```python
from build123d import *

# Parameters (mm, degrees)
F0_R     = 11.5
F0_R_2   = 5.5
F1_DEPTH = 1
F0_R_3   = 4.05
F2_DEPTH = 2
F0_R_4   = 2
F3_DEPTH = 5


# Not quite as in the source:
# - a fillet or chamfer that OpenCascade refuses, or shapes differently, is made with other operations: its cross-section is extruded or revolved along the edge and cut away or added


with BuildPart() as f1:
    # F0 (on Top) → F1 (new body)
    with BuildSketch(Plane.XY):
        Circle(F0_R)
        Circle(F0_R_2, mode=Mode.SUBTRACT)
    extrude(amount=F1_DEPTH)

    # F0 (on Top) → F2 (join)
    with BuildSketch(Plane.XY):
        Circle(F0_R_2)
        Circle(F0_R_3, mode=Mode.SUBTRACT)
    extrude(amount=F2_DEPTH)

    # F0 (on Top) → F3 (join)
    with BuildSketch(Plane.XY):
        Circle(F0_R_3)
        Circle(F0_R_4, mode=Mode.SUBTRACT)
        Circle(F0_R_4)
    extrude(amount=F3_DEPTH)

    # F4: fillet of radius 2 on 1 edges, made by hand

    # F4_s1 → F4_t2 (revolve, cut)
    with BuildSketch(Plane.XZ):
        with BuildLine():
            ThreePointArc((11.5, 1), (10.7679491924, 0.2679491924), (9.7679491924, 0))
            Line((9.7679491924, 0), (11.5, 0))
            Line((11.5, 0), (11.5, 1))
        make_face()
    revolve(axis=Axis((0, 0, 0), (0, 0, 1)), mode=Mode.SUBTRACT)


solid = f1.part
```
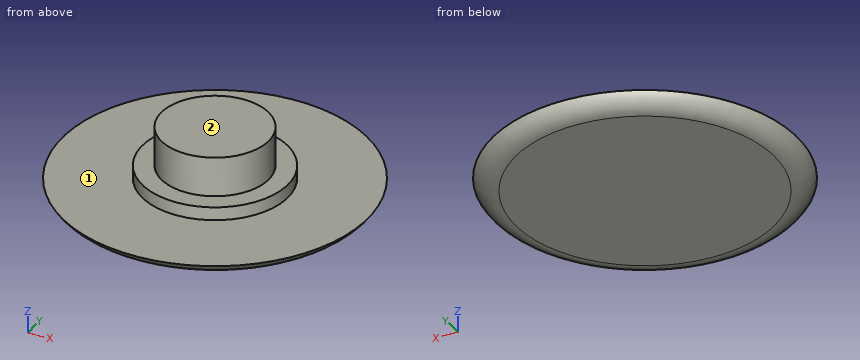
Geometry: final body of the model. Coordinates: model frame, mm. Face numbers are marked on the shaded views. A direction names the side the tool comes from. Coordinates: 2 decimals unless noted, no trailing zeros. Order: outer loops, then holes, each group sorted by start corner. A loop starts at its lowest first (then second) coordinate and runs counter-clockwise, first axis right, second up. Notation, with made-up numbers: (-7.75, 40.5) - (12.25, 40.5) arc R16 ccw to (12.25, 54.5) - close; hole circle Ø9 at (-1.75, 46.5). An arc over 180 degrees is marked (long way). Write each question's results on one line, items separated by ' | '.
1) Section C-C, the plane z = 2.8. Return loops of the section in (x, y), plus the area to 3 significant figures.
Results list:
outline: circle Ø8.1 at (0, 0) | area: 51.5 mm^2
2) Pin query (flat end, axial travel): pin 1 (3 mm diameter, centred on y = -1, z = 3, fed in from -X); pin 2 (1 mm diameter, centred on x = 3, z = 3.5, fed in from +Y); pin 3 (4 mm diameter, centred on x = -9, y = 6, fed in from +Z). Return the tip coordinate at first contact, or that it passes through.
Results list:
pin 1: x = -5.5 | pin 2: y = 3.19 | pin 3: z = 1
3) Section A-A, the plane y = 0. Return loops of the section in (x, z), plus the area to 3 significant figures.
Results list:
outline: (-11.5, 1) arc R2 ccw to (-9.77, 0) - (9.77, 0) arc R2 ccw to (11.5, 1) - (5.5, 1) - (5.5, 2) - (4.05, 2) - (4.05, 5) - (-4.05, 5) - (-4.05, 2) - (-5.5, 2) - (-5.5, 1) - close | area: 57.3 mm^2
4) Section D-D, the plane z = 0.6. Return loops of the section in (x, y), plus the area to 3 significant figures.
Results list:
outline: circle Ø22.39 at (0, 0) | area: 394 mm^2
5) Set-up query: the marked faces 1 and 2. Return all of +Z, -Z, +X, -X, +Y, -Y with unobstructed straight access to the full face (end or side cutting, diameter ignored); none if empty.
Results list:
face 1: +Z | face 2: +Z, +X, -X, +Y, -Y
6) Line query: line 1 (Z direction, x = 6.5, y = -1); line 2 (Y direction, x = 8.25, z = 0.7); line 3 (X direction, y = 3.25, z = 3.2). Output: solid intervals per line, ascending. Write a range as from..to.
Results list:
line 1: 0..1 | line 2: -7.7..7.7 | line 3: -2.42..2.42
